CAD build for the part. Positions are in the model's coordinates, mm. A direction names the side the tool comes from. Give positions to 0.01 mm unless a question says otherwise; leave off trailing zeros. Write each loop counter-clockwise with the first axis right and the second up, starting at its lowest first coordinate (ties: lowest second). Pieces come first, ordered by that corner, then holes. Notation, with made-up numbers: (57, 18) - (69, 18) arc R23 ccw to (69, 30) - close; hole circle Ø11 at (46.25, 63). An arc over 180 degrees is marked (long way). Put each result on its own line as item: value. Start each with the question number.
1. Cut at C-C on y = 5.25. List the corners of the cut face in (x, z), and give its area (3 significant figures).
2. Tool access for faces 4 (the flat face through (-3, 11, 15)), 5 (the flat face through (4, 3.5, 25)), 6 (the flat face through (3.603, 11.126, 22.912)), 7 (the flat face through (-2, 17, 11.65)), 8 (the cylindrical face through (4.466, 11.126, 23.4)): list every direction of +Z, -Z, +X, -X, +Y, -Y with a clear straight run to the whole face (end or side of a thin tool).
3. Cut at D-D on y = 19. List the corners of the cut face in (x, z).
4. Mould opens along Y. For faces 1 (the flat face through (1.84, 11.13, 6.37)), 2 (the flat face through (-4, 11, 9.15)), 3 (the flat face through (-1.2, 2, 15)) say: +Y half, -Y half, draft (parallel to the pull), parting line (faces both ways), or undercut.
5. Cut at B-B on z = 12.5. List the corners of the cut face in (x, y).
6. Wall check: line 1 (Y direction, x = -4.5, z = 13.75); line 2 (X direction, y = 13, z = 14.75); line 3 (Z direction, x = 1, y = 9.75). Give the ranges that are in metal, low to high.
7. Drop flat-ended pins along their axis: pin 1 (2 mm diameter, centred on x = 2, z = 17, fed in from +Y); pin 2 (0.9 mm diameter, centred on x = -3.5, y = 12.5, fed in from -Z); pin 3 (1.3 mm diameter, centred on x = -3.5, y = 11, fed in from +Z); pin 4 (1.6 mm diameter, centred on x = -3.5, y = 17.5, fed in from +Z). Give the stop position or say it passes through.
8. Cut at A-A on y = 15. List the corners of the cut face in (x, z).
from build123d import *

# Parameters (mm, degrees)
BOSS_EXTRUDE1_DEPTH      = 30.3
CUT_EXTRUDE1_DEPTH       = 181.717957049
CUT_EXTRUDE7_DEPTH       = 27.29
CUT_EXTRUDE10_DEPTH      = 96
CUT_EXTRUDE11_DEPTH      = 48
SKETCH9_W                = 2
SKETCH9_H                = 7.4
BOSS_EXTRUDE2_DEPTH      = 1.5
FILLET8_R                = 1
CUT_EXTRUDE15_DEPTH      = 2.6
CUT_EXTRUDE15_DEPTH_BACK = 2.6
SKETCH10_W               = 29
SKETCH10_H               = 15.5
SKETCH11_W               = 3.45
SKETCH11_H               = 8
BOSS_EXTRUDE3_DEPTH      = 1.3
FILLET9_R                = 7
CUT_EXTRUDE18_DEPTH      = 2.5
CUT_EXTRUDE23_START      = -2.5
CUT_EXTRUDE23_DEPTH      = 2.5
SKETCH18_W               = 4.5
SKETCH18_H               = 15
SKETCH18_W_2             = 3.45
SKETCH18_H_2             = 8
CUT_EXTRUDE24_DEPTH      = 1
THICKEN1_START           = 2
THICKEN1_DEPTH           = 168
CUT_EXTRUDE25_DEPTH      = 174.737489032
CUT_EXTRUDE25_DEPTH_BACK = 174.737489032
SKETCH20_W               = 39.19521875
SKETCH20_H               = 150
CUT_EXTRUDE27_DEPTH      = 2
SKETCH21_3_W             = 7
SKETCH21_3_H             = 2
CUT_EXTRUDE28_DEPTH      = 30.97192195
SKETCH22_W               = 8
SKETCH22_H               = 18
CUT_EXTRUDE29_DEPTH      = 30.97192195
BOSS_EXTRUDE4_DEPTH      = 18
SKETCH27_W               = 1.5
SKETCH27_H               = 15


# Read off the part's stored shape, not the designer's step: Cut-Extrude23, Thicken1
# Some blends are built 0.0001 mm under size
with BuildPart() as part:
    # Sketch1 → Boss-Extrude1 (new body)
    with BuildSketch(Plane.XY):
        Polygon((34.45, 2), (35.7, 0), (53.3, 0), (53.3, 48), (45, 74), (45, 170), (0, 170), (0, 2), align=None)
    extrude(amount=BOSS_EXTRUDE1_DEPTH)

    # Sketch2 → Cut-Extrude1 (cut, through all)
    with BuildSketch(Plane(origin=(0, 170, 0), x_dir=(1, 0, 0), z_dir=(0, 1, 0))):
        with BuildLine():
            Line((0, -30.3), (9.25, -30.3))
            ThreePointArc((9.25, -30.3), (2.495291793, -24.025316905), (0, -15.150000022))
            Line((0, -15.150000022), (0, -30.3))
        make_face()
        with BuildLine():
            ThreePointArc((0, -15.150000022), (2.495291781, -6.274683113), (9.25, 0))
            Line((9.25, 0), (0, 0))
            Line((0, 0), (0, -15.150000022))
        make_face()
    extrude(amount=-CUT_EXTRUDE1_DEPTH, mode=Mode.SUBTRACT)

    # Sketch7 → Cut-Extrude7 (cut)
    with BuildSketch(Plane(origin=(-8.97657775, 28.11940018, 0), x_dir=(0, 0, -1), z_dir=(0.30411092373144827, -0.9526366285563479, 0))):
        with BuildLine():
            Line((-15.15, 65.372856641), (-30.3, 65.372856641))
            Line((-30.3, 65.372856641), (-30.3, 56.120928382))
            ThreePointArc((-30.3, 56.120928382), (-24.02581935, 62.876979624), (-15.15, 65.372856641))
        make_face()
        with BuildLine():
            Line((0, 65.372856641), (-15.15, 65.372856641))
            ThreePointArc((-15.15, 65.372856641), (-6.27418065, 62.876979624), (0, 56.120928382))
            Line((0, 56.120928382), (0, 65.372856641))
        make_face()
    extrude(amount=-CUT_EXTRUDE7_DEPTH, mode=Mode.SUBTRACT)

    # Sketch6 → Cut-Extrude10 (cut)
    with BuildSketch(Plane(origin=(0, 170, 0), x_dir=(1, 0, 0), z_dir=(0, 1, 0))):
        with BuildLine():
            Line((45, -15.15), (45, 0))
            Line((45, 0), (35.74807174, 0))
            ThreePointArc((35.74807174, 0), (42.504122982, -6.27418065), (45, -15.15))
        make_face()
        with BuildLine():
            Line((45, -30.3), (45, -15.15))
            ThreePointArc((45, -15.15), (42.504122982, -24.02581935), (35.74807174, -30.3))
            Line((35.74807174, -30.3), (45, -30.3))
        make_face()
    extrude(amount=-CUT_EXTRUDE10_DEPTH, mode=Mode.SUBTRACT)

    # Sketch4 → Cut-Extrude11 (cut)
    with BuildSketch(Plane.XZ):
        with BuildLine():
            Line((53.3, 15.15), (53.3, 30.3))
            Line((53.3, 30.3), (44.04807174, 30.3))
            ThreePointArc((44.04807174, 30.3), (50.804122982, 24.02581935), (53.3, 15.15))
        make_face()
        with BuildLine():
            Line((53.3, 0), (53.3, 15.15))
            ThreePointArc((53.3, 15.15), (50.804122982, 6.27418065), (44.04807174, 0))
            Line((44.04807174, 0), (53.3, 0))
        make_face()
    extrude(amount=-CUT_EXTRUDE11_DEPTH, mode=Mode.SUBTRACT)

    # Sketch9 → Boss-Extrude2 (add)
    with BuildSketch(Plane.XZ.offset(-2)):
        with Locations((3, 15.15)):
            Rectangle(SKETCH9_W, SKETCH9_H)
    extrude(amount=BOSS_EXTRUDE2_DEPTH)

    # Fillet8
    fillet8_edges = [part.edges().sort_by_distance(p)[0] for p in [
        (4, 1.25, 11.45),
        (2, 1.25, 11.45),
        (4, 1.25, 18.85),
        (2, 1.25, 18.85),
    ]]
    fillet(fillet8_edges, radius=FILLET8_R - 0.0001)  # a hair under: the kernel refuses the full size

    # Sketch10 → Cut-Extrude15 (cut, two sides: drawn at the far end of the back side and taken through both)
    with BuildSketch(Plane.XZ.offset(-2).offset(-CUT_EXTRUDE15_DEPTH_BACK)):
        with Locations((21, 15.15)):
            Rectangle(SKETCH10_W, SKETCH10_H)
    extrude(amount=CUT_EXTRUDE15_DEPTH + CUT_EXTRUDE15_DEPTH_BACK, mode=Mode.SUBTRACT)

    # Sketch11 → Boss-Extrude3 (add)
    with BuildSketch(Plane.XZ):
        with Locations((43.575, 15.15)):
            Rectangle(SKETCH11_W, SKETCH11_H)
    extrude(amount=BOSS_EXTRUDE3_DEPTH)

    # Fillet9
    # the kernel refuses this fillet: 7 mm, written as the material it takes off along each edge
    with BuildSketch(Plane(origin=(55.458124827, -1.3, 11.15), x_dir=(0, 1, 0), z_dir=(-1, 0, 0)), Plane(origin=(31.691875173, -1.3, 19.15), x_dir=(0, 1, 0), z_dir=(1, 0, 0))) as fillet9_piece_1:
        with BuildLine():
            CenterArc((7, -4.063249931), FILLET9_R, 144.516796045, 35.483203955)
            Line((0, -4.063249931), (-0.14, -4.063249931))
            Line((-0.14, -4.063249931), (-0.14, 0))
            Line((-0.14, 0), (0, 0.14))
            ThreePointArc((0, 0.14), (0.65, 0.14), (1.186, 0.081264999))
            Line((1.186, 0.081264999), (1.3, 0))
        make_face()
    extrude(amount=23.766249654, mode=Mode.SUBTRACT)

    # Sketch13 → Cut-Extrude18 (cut)
    with BuildSketch(Plane(origin=(0, 74, 0), x_dir=(1, 0, 0), z_dir=(0, 1, 0))):
        with BuildLine():
            Line((35.74807174, -30.3), (45, -30.3))
            Line((45, -30.3), (45, -15.15))
            ThreePointArc((45, -15.15), (42.504122982, -24.02581935), (35.74807174, -30.3))
        make_face()
    extrude(amount=-CUT_EXTRUDE18_DEPTH, mode=Mode.SUBTRACT)

    # Cut-Extrude23 outline → Cut-Extrude23 (cut)
    with BuildSketch(Plane(origin=(0, 74, 0), x_dir=(1, 0, 0), z_dir=(0, 1, 0)).offset(CUT_EXTRUDE23_START)):
        with BuildLine():
            ThreePointArc((44.999624541, -15.036915931), (44.999829684, -15.061319249), (45, -15.085722835))
            Line((45, -15.085722835), (45, 0))
            Line((45, 0), (35.74807174, 0))
            ThreePointArc((35.74807174, 0), (42.474573722, -6.225973939), (44.999624541, -15.036915931))
        make_face()
    extrude(amount=CUT_EXTRUDE23_DEPTH, mode=Mode.SUBTRACT)

    # Sketch18 → Cut-Extrude24 (cut)
    with BuildSketch(Plane.XZ):
        with Locations((43.575, 15.15)):
            Rectangle(SKETCH18_W, SKETCH18_H)
        with Locations((43.575, 15.15)):
            Rectangle(SKETCH18_W_2, SKETCH18_H_2, mode=Mode.SUBTRACT)
    extrude(amount=-CUT_EXTRUDE24_DEPTH, mode=Mode.SUBTRACT)


with BuildPart() as body_2:
    # Thicken1 outline → Thicken1 (new body)
    with BuildSketch(Plane(origin=(0, 0, 0), x_dir=(1, 0, 0), z_dir=(0, 1, 0)).offset(THICKEN1_START)):
        with BuildLine():
            Line((8.793107415, 0.889521875), (6.965537077, 4.447609375))
            ThreePointArc((6.965537077, 4.447609375), (-5, -15.15), (6.965537077, -34.747609375))
            Line((6.965537077, -34.747609375), (8.793107415, -31.189521875))
            ThreePointArc((8.793107415, -31.189521875), (-1, -15.15), (8.793107415, 0.889521875))
        make_face()
    extrude(amount=THICKEN1_DEPTH)

    # Sketch20 → Cut-Extrude25 (cut, two sides: drawn at the far end of the back side and taken through both)
    with BuildSketch(Plane(origin=(0, 0, 0), x_dir=(0, 0, -1), z_dir=(1, 0, 0)).offset(-CUT_EXTRUDE25_DEPTH_BACK)):
        with Locations((-15.15, 95)):
            Rectangle(SKETCH20_W, SKETCH20_H)
    extrude(amount=CUT_EXTRUDE25_DEPTH + CUT_EXTRUDE25_DEPTH_BACK, mode=Mode.SUBTRACT)

    # Sketch21 → Cut-Extrude27 (cut)
    with BuildSketch(Plane(origin=(-5, 20, 15.15), x_dir=(0, 0, 1), z_dir=(-1, 0, 0))):
        Polygon((-3.5, -3), (-6, -3), (-6, -9), (6, -9), (6, -3), (3.5, -3), (3.5, -4), (-3.5, -4), align=None)
        Polygon((6, -9), (-6, -9), (-6, -15), (-3.5, -15), (-3.5, -14), (3.5, -14), (3.5, -15), (6, -15), align=None)
    extrude(amount=-CUT_EXTRUDE27_DEPTH, mode=Mode.SUBTRACT)

    # Sketch21<3> → Cut-Extrude28 (cut, through all)
    with BuildSketch(Plane(origin=(-5, 20, 15.15), x_dir=(0, 0, 1), z_dir=(-1, 0, 0))):
        with Locations((0, -3)):
            Rectangle(SKETCH21_3_W, SKETCH21_3_H)
        with Locations((0, -15)):
            Rectangle(SKETCH21_3_W, SKETCH21_3_H)
    extrude(amount=-CUT_EXTRUDE28_DEPTH, mode=Mode.SUBTRACT)

    # Sketch22 → Cut-Extrude29 (cut, through all)
    with BuildSketch(Plane(origin=(-5, 20, 15.15), x_dir=(0, 0, 1), z_dir=(-1, 0, 0))):
        with Locations((15.597609375, -9)):
            Rectangle(SKETCH22_W, SKETCH22_H)
        with Locations((-15.597609375, -9)):
            Rectangle(SKETCH22_W, SKETCH22_H)
    extrude(amount=-CUT_EXTRUDE29_DEPTH, mode=Mode.SUBTRACT)

    # Sketch26 → Boss-Extrude4 (add, through all)
    with BuildSketch(Plane(origin=(0, 20, 0), x_dir=(1, 0, 0), z_dir=(0, 1, 0))):
        with BuildLine():
            ThreePointArc((1.420420678, -24.173845266), (2.266305947, -25.500112624), (3.224564184, -26.747609375))
            Line((3.224564184, -26.747609375), (5.521704906, -24.818064221))
            ThreePointArc((5.521704906, -24.818064221), (4.722876296, -23.778118977), (4.01772467, -22.672508539))
            Line((4.01772467, -22.672508539), (1.420420678, -24.173845266))
        make_face()
        with BuildLine():
            Line((5.521704906, -5.481935779), (3.224564184, -3.552390625))
            ThreePointArc((3.224564184, -3.552390625), (2.266305947, -4.799887376), (1.420420678, -6.126154734))
            Line((1.420420678, -6.126154734), (4.01772467, -7.627491461))
            ThreePointArc((4.01772467, -7.627491461), (4.722876296, -6.521881023), (5.521704906, -5.481935779))
        make_face()
    extrude(amount=-BOSS_EXTRUDE4_DEPTH)

    # Sketch27 → Cut-Revolve1 (revolve, cut)
    with BuildSketch(Plane(origin=(14.50695613, 0, 17.270660706), x_dir=(0.765713574037014, 0, -0.6431817181290699), z_dir=(0.6431817181290699, 0, 0.765713574037014))):
        with Locations((-13.234480788, 11)):
            Rectangle(SKETCH27_W, SKETCH27_H)
    revolve(axis=Axis((17.031621622, 2, 15.15), (0, 1, 0)), mode=Mode.SUBTRACT)

    # Chamfer1
    # the kernel refuses this chamfer: 1 mm, written as the material it takes off along each edge
    with BuildSketch(Plane(origin=(5.521704906, 22.495775164, 5.481935779), x_dir=(-0.5957324474314561, 0, 0.8031829499418718), z_dir=(0, -1, 0))) as chamfer1_piece_1:
        with BuildLine():
            Line((0.966778181, 0), (-0.087645206, 0.994455281))
            Line((-0.087645206, 0.994455281), (-0.107608652, 0.993246637))
            ThreePointArc((-0.107608652, 0.993246637), (-0.050117113, 0.496846553), (-0.019963446, -0.001208643))
            Line((-0.019963446, -0.001208643), (0.001208643, -0.019963446))
            ThreePointArc((0.001208643, -0.019963446), (0.48334789, 0.001454531), (0.966739217, -0.019999962))
            Line((0.966739217, -0.019999962), (0.966778181, 0))
        make_face()
    extrude(amount=22.991550328, mode=Mode.SUBTRACT)
    with BuildSketch(Plane(origin=(5.521704906, 22.495775164, 24.818064221), x_dir=(-0.7477801322117752, 0, 0.6639464390064458), z_dir=(0, -1, 0))) as chamfer1_piece_2:
        with BuildLine():
            Line((0.998310066, 0), (-0.084876909, 0.96304515))
            Line((-0.084876909, 0.96304515), (-0.104796224, 0.961250468))
            ThreePointArc((-0.104796224, 0.961250468), (-0.040985923, 0.481609232), (-0.019992472, -0.000548686))
            Line((-0.019992472, -0.000548686), (0.000548686, -0.019992472))
            ThreePointArc((0.000548686, -0.019992472), (0.499328034, -0.006303662), (0.998858751, -0.019992472))
            Line((0.998858751, -0.019992472), (0.998310066, 0))
        make_face()
    extrude(amount=22.991550328, mode=Mode.SUBTRACT)


solid = body_2.part
Report:
1. outline: (-4.17, 9.15) arc R22.03 ccw to (-1.7, 3.55) - (3.22, 3.55) - (3.8, 4.03) arc R17.28 cw to (2.07, 6.5) - (1.42, 6.13) arc R18.03 cw to (-0.66, 11.65) - (-3, 11.65) - (-3, 9.15) - close; (-4.17, 21.15) - (-3, 21.15) - (-3, 18.65) - (-0.66, 18.65) arc R18.03 cw to (1.42, 24.17) - (2.07, 23.8) arc R17.28 cw to (3.8, 26.27) - (3.22, 26.75) - (-1.7, 26.75) arc R22.03 ccw to start; (3.37, 7.25) arc R15.78 ccw to (4.82, 5.16) - (4.94, 6.22) arc R15.03 cw to (4.02, 7.63) - close; (3.37, 23.05) - (4.02, 22.67) arc R15.03 cw to (4.94, 24.08) - (4.82, 25.14) arc R15.78 ccw to start
1. area: 71.4 mm²
2. face 4: -X
2. face 5: none
2. face 6: +Y, -Y
2. face 7: +X, -X
2. face 8: +X, +Y, -Y
3. outline: (-1.7, 3.55) - (3.22, 3.55) - (4.78, 4.86) - (4.94, 6.22) arc R15.03 cw to (4.02, 7.63) - (1.42, 6.13) arc R18.03 cw to (1.42, 24.17) - (4.02, 22.67) arc R15.03 cw to (4.94, 24.08) - (4.78, 25.44) - (3.22, 26.75) - (-1.7, 26.75) arc R22.03 ccw to start
4. face 1: draft
4. face 2: undercut
4. face 3: -Y half
5. outline: (-4.84, 2) - (-0.8, 2) - (-0.8, 4) - (-4.84, 4) - close; (-4.84, 18) - (-0.8, 18) - (-0.8, 20) - (-4.84, 20) - close; (-3, 6) - (-0.8, 6) - (-0.8, 16) - (-3, 16) - close
6. line 1: y = 2 to 4, 18 to 20
6. line 2: x = -3 to -1
6. line 3: z = 3.55 to 6.9, 23.4 to 26.75
7. pin 1: passes through
7. pin 2: stops at z = 6.09
7. pin 3: stops at z = 24.64
7. pin 4: stops at z = 24.95
8. outline: (-4.17, 9.15) arc R22.03 ccw to (-1.7, 3.55) - (3.22, 3.55) - (3.8, 4.03) arc R17.28 cw to (2.07, 6.5) - (1.42, 6.13) arc R18.03 cw to (1.42, 24.17) - (2.07, 23.8) arc R17.28 cw to (3.8, 26.27) - (3.22, 26.75) - (-1.7, 26.75) arc R22.03 ccw to (-4.17, 21.15) - (-3, 21.15) - (-3, 9.15) - close; (3.37, 7.25) arc R15.78 ccw to (4.82, 5.16) - (4.94, 6.22) arc R15.03 cw to (4.02, 7.63) - close; (3.37, 23.05) - (4.02, 22.67) arc R15.03 cw to (4.94, 24.08) - (4.82, 25.14) arc R15.78 ccw to start
